For this review, take the finished solid that the model builds, in its own axes (mm). A direction names the side the tool comes from. Give positions to 0.01 mm unless a question says otherwise; leave off trailing zeros. Order: outer loops, then holes, each group sorted by start corner. A loop starts at its lowest first (then second) coordinate and runs counter-clockwise, first axis right, second up.
Item 1: For P1, Ø0.8, axis at x = 1, y = -12, coming from the +Z side; P2, Ø2, axis at y = -5.5, z = 0, coming from the +X side; P3, Ø1.2, axis at y = -8, z = 1, coming from the +X side; P4, Ø1.5, axis at x = 0, z = 0, coming from the +Y side, all flat-tipped, find the tip position at first contact; note any pin that passes through.
Item 2: Consider section A-A (y = -4). Give the boundary of the cut face in (x, z), plus the area to 3 significant figures.
Item 3: The part is to be moulded in two halves that separate along X. For faces 4 (the cylindrical face through (0.28, -9.28, 0.53)), 5 (the cylindrical face through (-0.29, -2.66, 2.23)), 6 (the flat face through (1, -10, 0.125)), say which applies: released by +X, released by -X, zero draft, split by the parting line, or undercut.
Item 4: For probe 1 along Z at (x, y) = (0, -2.1); probe 2 along X at (y, z) = (-8.75, 0.3); probe 3 along X at (y, z) = (-7, -1.3) (3 decimals), list the stretches that pass through material, from the lowest coordinate up.
Item 5: Machinability: for faces 1 (the flat face through (1, 0, 1)), 2 (the flat face through (-1, -10, -0.125)), 3 (the flat face through (0.125, -10, -1)), which of the approach directions +Z, -Z, +X, -X, +Y, -Y give a long, thin tool a straight path to every point of the face, cutting with its end or side? Answer none if there is none.
Autodesk Inventor part; units mm, degrees
ref_plane "YZ Plane" through (0, 0, 0) normal (1, 0, 0) x (0, 1, 0)
ref_plane "XZ Plane" through (0, 0, 0) normal (0, 1, 0) x (-1, 0, 0)
ref_plane "XY Plane" through (0, 0, 0) normal (0, 0, 1) x (1, 0, 0)
sketch "Sketch1" plane through (0, 0, 0) normal (0, 0, 1) x (1, 0, 0)
  line L0 (0, 0) -> (0, -5.8)
  line L1 (0, 0) -> (2.25, 0)
  line L2 (2.25, 0) -> (2.25, -5)
  line L3 (2.25, -5) -> (1.5, -5)
  line L4 (1.5, -5) -> (1.5, -14.7)
  line L5 (1.5, -14.7) -> (0.7, -14.7)
  line L6 (0.7, -14.7) -> (0.45, -14.45)
  line L7 (0.45, -14.45) -> (0.45, -13.95)
  line L8 (0.45, -13.95) -> (0.6, -13.8)
  line L9 (0.6, -13.8) -> (0.6, -5.8)
  line L10 (0.6, -5.8) -> (0, -5.8)
  line L11 (1, -14.7) -> (1.5, -5.5)
  line L12 (0.6, -5.8) -> (0.6, 0)
  dimension "d0" = 4.5
  dimension "d1" = 0.9
  dimension "d2" = 1.2
  dimension "d3" = 135
  dimension "d4" = 3
  dimension "d5" = 5
  dimension "d6" = 0.8
  dimension "d7" = 8
  dimension "d8" = 0.25
  dimension "d9" = 0.5
  dimension "d10" = 0.5
  dimension "d11" = 0.3
revolve "Revolution1" add sketch "Sketch1" angle 360 about axis through (0, 0, 0) along (0, -1, 0) contours L1 L2 L3 L4 L11 L5 L6 L7 L8 L9 L12
sketch "Sketch3" plane through (0, 0, 0) normal (0, 1, 0) x (1, 0, 0)
  circle A0 centre (0, 0) radius 0.6
hole "Hole1" at (0, 0, 0) direction (0, -1, 0) diameter 2.459 depth 4.5 tip angle 118
chamfer "Chamfer2" distance 0.25 angle 45 1 edges at (-2.25, 0, 0)
sketch "Sketch2" plane through (0, -14.7, 0) normal (0, -1, 0) x (1, 0, 0)
  line L0 (-0.125, -2.2191) -> (0.125, -2.2191)
  line L1 (0.125, -2.2191) -> (0.125, 2.2191)
  line L2 (0.125, 2.2191) -> (-0.125, 2.2191)
  line L3 (-0.125, 2.2191) -> (-0.125, -2.2191)
  line L4 (-0.125, -2.2191) -> (0.125, 2.2191) construction
  line L5 (0.125, -2.2191) -> (-0.125, 2.2191) construction
  line L6 (-2.0682, -0.125) -> (2.0682, -0.125)
  line L7 (2.0682, -0.125) -> (2.0682, 0.125)
  line L8 (2.0682, 0.125) -> (-2.0682, 0.125)
  line L9 (-2.0682, 0.125) -> (-2.0682, -0.125)
  line L10 (-2.0682, -0.125) -> (2.0682, 0.125) construction
  line L11 (2.0682, -0.125) -> (-2.0682, 0.125) construction
  point P0 (0, 0)
  point P1 (-0.125, -0.125)
  point P2 (0.125, -0.125)
  point P3 (0.125, 0.125)
  point P4 (-0.125, 0.125)
  dimension "d13" = 0.25
  dimension "d14" = 0.25
extrude "Extrusion1" cut sketch "Sketch2" against normal blind 9
chamfer "Chamfer3" distance 0.5 angle 45 1 edges at (-1.5, -5, 0)
equation "\"d13\" = d14"
properties part number "FilamentPin" material "Copper"
Resolved:
1. P1: stops at z = 0.98
1. P2: stops at x = 2.25
1. P3: stops at x = 1.31
1. P4: stops at y = -4.79
2. outline: circle Ø4.5 at (0, 0); hole circle Ø2.46 at (0, 0)
2. area: 11.2 mm2
3. face 4: undercut
3. face 5: split by the parting line
3. face 6: zero draft
4. probe 1: z = -2.25 to -1.23, 1.23 to 2.25
4. probe 2: x = -1.29 to -0.52, 0.52 to 1.29
4. probe 3: x = -0.568 to -0.125, 0.125 to 0.568
5. face 1: +Z, -Z, +X, -X, +Y
5. face 2: +X, -X, -Y
5. face 3: +Z, -Z, -Y
